```python
from build123d import *

# Parameters (mm, degrees)
SKETCH1_R           = 3.75
BOSS_EXTRUDE1_DEPTH = 5
SKETCH2_R           = 5
BOSS_EXTRUDE2_DEPTH = 2
BOSS_EXTRUDE3_DEPTH = 16.6
SKETCH4_R           = 3.204293994
BOSS_EXTRUDE4_DEPTH = 7


with BuildPart() as part:
    # Sketch1 → Boss-Extrude1 (new body)
    with BuildSketch(Plane.XY):
        Circle(SKETCH1_R)
    extrude(amount=BOSS_EXTRUDE1_DEPTH)

    # Sketch2 → Boss-Extrude2 (add)
    with BuildSketch(Plane.XY.offset(5)):
        Circle(SKETCH2_R)
    extrude(amount=BOSS_EXTRUDE2_DEPTH)

    # Sketch3 → Boss-Extrude3 (add)
    with BuildSketch(Plane.XY.offset(7)):
        Polygon((3.7, 0), (1.85, 3.204293994), (-1.85, 3.204293994), (-3.7, 0), (-1.85, -3.204293994), (1.85, -3.204293994), align=None)
    extrude(amount=BOSS_EXTRUDE3_DEPTH)

    # Sketch4 → Boss-Extrude4 (add)
    with BuildSketch(Plane.XY.offset(23.6)):
        Circle(SKETCH4_R)
    extrude(amount=BOSS_EXTRUDE4_DEPTH)


solid = part.part
```
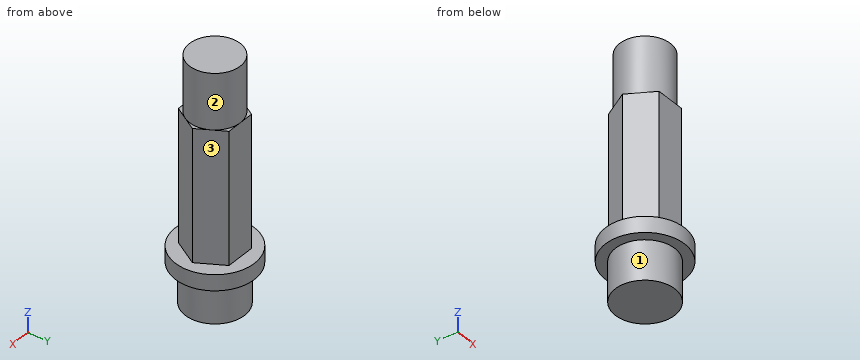
The listing builds one solid part. Answer for the finished solid, in the listing's coordinates (mm). Face numbers are marked on the shaded views. A direction names the side the tool comes from. Give positions to 0.01 mm unless a question says otherwise; leave off trailing zeros. Order: outer loops, then holes, each group sorted by start corner. A loop starts at its lowest first (then second) coordinate and runs counter-clockwise, first axis right, second up. Notation, with made-up numbers: (-39, 21) -> (-10, 21) arc R28 ccw to (-10, 47) -> close; hole circle Ø7 at (-15, 14). An arc over 180 degrees is marked (long way). Answer as a JSON object with one key per item and string values. Group by question number.
Item 1: The part is cut by section B-B on z = 27.5. Write down the section's boundary in (x, y).
Item 2: A tool of negligible diameter and unlimited length cuts with its end or side. For the marked faces 1, 2 and 3, from which of +Z, -Z, +X, -X, +Y, -Y can it reach the whole face along a straight path? Write none if from no direction.
Item 3: Flat-ended cylindrical pins translate along their axes: pin 1 (3 mm diameter, centred on x = 3.5, z = 7, fed in from -Y); pin 2 (2 mm diameter, centred on y = -3.5, z = 16.5, fed in from +X); pin 3 (5 mm diameter, centred on y = -1.5, z = 25, fed in from +X). Find the tip coordinate at first contact, or state that the pin passes through.
Item 4: Consider L1, parallel to X at y = 0.25, z = 6; L2, parallel to Y at x = 0, z = 21; L3, parallel to Z at x = -2, y = 3.5. Determine where each line is inside the solid, lowest interval first. Write a range as from..to.
Item 5: The part is cut by section A-A on y = -0.75. Write down the section's boundary in (x, z), and give its area (3 significant figures).
Item 6: The part is cut by section D-D on x = 4.25. Write down the section's boundary in (y, z), and give its area (3 significant figures).
Result set:
{
 "1": {"outline": "circle Ø6.41 at (0, 0)"},
 "2": {"face 1": "-Z", "face 2": "+Z", "face 3": "+Z, +X, +Y"},
 "3": {"pin 1": "y = -4.58", "pin 2": "x = 2.26", "pin 3": "x = 3.7"},
 "4": {"L1": "-4.99..4.99", "L2": "-3.2..3.2", "L3": "5..7"},
 "5": {"outline": "(-4.94, 5) -> (-3.67, 5) -> (-3.67, 0) -> (3.67, 0) -> (3.67, 5) -> (4.94, 5) -> (4.94, 7) -> (3.27, 7) -> (3.27, 23.6) -> (3.12, 23.6) -> (3.12, 30.6) -> (-3.12, 30.6) -> (-3.12, 23.6) -> (-3.27, 23.6) -> (-3.27, 7) -> (-4.94, 7) -> close", "area": "209 mm²"},
 "6": {"outline": "(-2.63, 5) -> (2.63, 5) -> (2.63, 7) -> (-2.63, 7) -> close", "area": "10.5 mm²"}
}
